from build123d import *

# Parameters (mm, degrees)
BASE_FLANGE1_DEPTH            = 1
EDGE_FLANGE1_STRIP_W          = 6
EDGE_FLANGE1_STRIP_H          = 1
EDGE_FLANGE1_STRIP_CUT_DEPTH  = 100
EDGE_FLANGE1_RELIEF_W         = 6.5
EDGE_FLANGE1_RELIEF_H         = 0.5
EDGE_FLANGE1_RELIEF_CUT_DEPTH = 1
EDGE_FLANGE1_DEPTH            = 100
EDGE_FLANGE1_PROFILE_W        = 100
EDGE_FLANGE1_PROFILE_H        = 19
EDGE_FLANGE1_PROFILE_R        = 1.5
EDGE_FLANGE1_FLAT_DEPTH       = 1
EDGE_FLANGE2_START            = 29.5
EDGE_FLANGE2_DEPTH            = 61
EDGE_FLANGE2_2_DEPTH          = 0.5
EDGE_FLANGE2_START_2          = 90
EDGE_FLANGE2_3_DEPTH          = 0.5
EDGE_FLANGE2_START_3          = 30
EDGE_FLANGE2_4_DEPTH          = 60
EDGE_FLANGE2_5_OUTLINE_R      = 1.5
EDGE_FLANGE2_5_DEPTH          = 1


with BuildPart() as part:
    # Base-Flange1: sheet metal written as solids
    # Sketch1 → Base-Flange1 (new body)
    with BuildSketch(Plane.XY):
        with BuildLine():
            Line((0, 0), (0, 350))
            Line((0, 350), (0, 375))
            ThreePointArc((0, 375), (-13.854151002, 365.75), (-27.708302005, 375))
            ThreePointArc((-27.708302005, 375), (-5.863059775, 415.921497754), (30, 386.5))
            Line((30, 386.5), (30, 346.5))
            Line((30, 346.5), (600, 280))
            Line((600, 280), (600, 0))
            Line((600, 0), (0, 0))
        make_face()
    extrude(amount=-BASE_FLANGE1_DEPTH)

    # Edge-Flange1: sheet metal written as solids
    # Edge-Flange1 strip (on a plane across the edge) → Edge-Flange1 strip cut (cut)
    with BuildSketch(Plane.YZ.offset(450)):
        with Locations((-1, -0.5)):
            Rectangle(EDGE_FLANGE1_STRIP_W, EDGE_FLANGE1_STRIP_H)
    edge_flange1_strip_cut = extrude(amount=EDGE_FLANGE1_STRIP_CUT_DEPTH, mode=Mode.SUBTRACT)

    # Edge-Flange1 relief (on the sheet) → Edge-Flange1 relief cut (cut)
    with BuildSketch(Plane(origin=(450, 2, 0), x_dir=(0, 1, 0), z_dir=(0, 0, 1))):
        with Locations((-2.75, 0.25)):
            Rectangle(EDGE_FLANGE1_RELIEF_W, EDGE_FLANGE1_RELIEF_H)
        with Locations((-2.75, -100.25)):
            Rectangle(EDGE_FLANGE1_RELIEF_W, EDGE_FLANGE1_RELIEF_H)
    edge_flange1_relief_cut = extrude(amount=-EDGE_FLANGE1_RELIEF_CUT_DEPTH, mode=Mode.SUBTRACT)

    # Edge-Flange1 bend section (on a plane across the edge) → Edge-Flange1 (add)
    with BuildSketch(Plane.YZ.offset(450)):
        with BuildLine():
            Line((0, 1), (1, 1))
            ThreePointArc((1, 1), (1.292893219, 0.292893219), (2, 0))
            Line((2, 0), (2, -1))
            ThreePointArc((2, -1), (0.585786438, -0.414213562), (0, 1))
        make_face()
    edge_flange1 = extrude(amount=EDGE_FLANGE1_DEPTH)

    # Edge-Flange1 profile (on flange) → Edge-Flange1 flat (add)
    with BuildSketch(Plane(origin=(0, 0, 0), x_dir=(-1, 0, 0), z_dir=(0, 1, 0))):
        with Locations((-500, 10.5)):
            Rectangle(EDGE_FLANGE1_PROFILE_W, EDGE_FLANGE1_PROFILE_H)
        with Locations((-535, 10)):
            Circle(EDGE_FLANGE1_PROFILE_R, mode=Mode.SUBTRACT)
        with Locations((-465, 10)):
            Circle(EDGE_FLANGE1_PROFILE_R, mode=Mode.SUBTRACT)
        with Locations((-500, 10)):
            Circle(EDGE_FLANGE1_PROFILE_R, mode=Mode.SUBTRACT)
    edge_flange1_flat = extrude(amount=EDGE_FLANGE1_FLAT_DEPTH)

    # Mirror1: Edge-Flange1 strip cut, Edge-Flange1 relief cut, Edge-Flange1, Edge-Flange1 flat across plane
    add(edge_flange1_strip_cut.mirror(Plane(origin=(300, 0, 0), x_dir=(0, 0, 1), z_dir=(1, 0, 0))), mode=Mode.SUBTRACT)
    add(edge_flange1_relief_cut.mirror(Plane(origin=(300, 0, 0), x_dir=(0, 0, 1), z_dir=(1, 0, 0))), mode=Mode.SUBTRACT)
    add(edge_flange1.mirror(Plane(origin=(300, 0, 0), x_dir=(0, 0, 1), z_dir=(1, 0, 0))))
    add(edge_flange1_flat.mirror(Plane(origin=(300, 0, 0), x_dir=(0, 0, 1), z_dir=(1, 0, 0))))

    # Edge-Flange2: read off the stored shape, not the designer's step
    # Edge-Flange2 outline → Edge-Flange2 (cut)
    with BuildSketch(Plane(origin=(0, 0, 0), x_dir=(1, 0, 0), z_dir=(0, 1, 0)).offset(EDGE_FLANGE2_START)):
        with BuildLine():
            ThreePointArc((0.363077531, 0), (1.095128339, 0.732050808), (2.095128339, 1))
            Line((2.095128339, 1), (0, 1))
            Line((0, 1), (0, 0))
            Line((0, 0), (0.363077531, 0))
        make_face()
    edge_flange2 = extrude(amount=EDGE_FLANGE2_DEPTH, mode=Mode.SUBTRACT)

    # Edge-Flange2 2 outline → Edge-Flange2 2 (cut)
    with BuildSketch(Plane(origin=(0, 0, 0), x_dir=(1, 0, 0), z_dir=(0, 1, 0)).offset(EDGE_FLANGE2_START)):
        with BuildLine():
            Line((2.595128339, 0), (2.595128339, 1))
            Line((2.595128339, 1), (2.095128339, 1))
            ThreePointArc((2.095128339, 1), (1.095128339, 0.732050808), (0.363077531, 0))
            Line((0.363077531, 0), (2.595128339, 0))
        make_face()
    edge_flange2_2 = extrude(amount=EDGE_FLANGE2_2_DEPTH, mode=Mode.SUBTRACT)

    # Edge-Flange2 3 outline → Edge-Flange2 3 (cut)
    with BuildSketch(Plane(origin=(0, 0, 0), x_dir=(1, 0, 0), z_dir=(0, 1, 0)).offset(EDGE_FLANGE2_START_2)):
        with BuildLine():
            Line((2.595128339, 0), (2.595128339, 1))
            Line((2.595128339, 1), (2.095128339, 1))
            ThreePointArc((2.095128339, 1), (1.095128339, 0.732050808), (0.363077531, 0))
            Line((0.363077531, 0), (2.595128339, 0))
        make_face()
    edge_flange2_3 = extrude(amount=EDGE_FLANGE2_3_DEPTH, mode=Mode.SUBTRACT)

    # Edge-Flange2 4 outline → Edge-Flange2 4 (add)
    with BuildSketch(Plane(origin=(0, 0, 0), x_dir=(1, 0, 0), z_dir=(0, 1, 0)).offset(EDGE_FLANGE2_START_3)):
        with BuildLine():
            ThreePointArc((1.098933641, -1.087155743), (1.357851002, -0.324409792), (2.095128339, 0))
            Line((2.095128339, 0), (0.363077531, 0))
            ThreePointArc((0.363077531, 0), (0.142536324, -0.567120772), (0.102738942, -1.174311485))
            Line((0.102738942, -1.174311485), (1.750739994, -20.011049705))
            Line((1.750739994, -20.011049705), (2.746934692, -19.923893962))
            Line((2.746934692, -19.923893962), (1.098933641, -1.087155743))
        make_face()
    edge_flange2_4 = extrude(amount=EDGE_FLANGE2_4_DEPTH)

    # Edge-Flange2 5 outline → Edge-Flange2 5 (cut)
    with BuildSketch(Plane(origin=(0, 0, 0), x_dir=(0, 1, 0), z_dir=(0.9961946980917459, 0, -0.0871557427476548))):
        with Locations((80, 10.087488664)):
            Circle(EDGE_FLANGE2_5_OUTLINE_R)
        with Locations((60, 10.087488664)):
            Circle(EDGE_FLANGE2_5_OUTLINE_R)
        with Locations((40, 10.087488664)):
            Circle(EDGE_FLANGE2_5_OUTLINE_R)
    edge_flange2_5 = extrude(amount=EDGE_FLANGE2_5_DEPTH, mode=Mode.SUBTRACT)

    # Mirror2: Edge-Flange2, Edge-Flange2 2, Edge-Flange2 3, Edge-Flange2 4, Edge-Flange2 5 across plane
    add(edge_flange2.mirror(Plane.ZX.offset(161.81)), mode=Mode.SUBTRACT)
    add(edge_flange2_2.mirror(Plane.ZX.offset(161.81)), mode=Mode.SUBTRACT)
    add(edge_flange2_3.mirror(Plane.ZX.offset(161.81)), mode=Mode.SUBTRACT)
    add(edge_flange2_4.mirror(Plane.ZX.offset(161.81)))
    add(edge_flange2_5.mirror(Plane.ZX.offset(161.81)), mode=Mode.SUBTRACT)


solid = part.part
Read the model definition and answer for the solid it produces. Units are mm, in the model's axes. A direction names the side the tool comes from. Round coordinates to 2 decimals unless told otherwise and drop trailing zeros. Write each loop counter-clockwise with the first axis right and the second up, starting at its lowest first coordinate (ties: lowest second). Pieces come first, ordered by that corner, then holes. Notation, with made-up numbers: (48.25, 14) - (61.25, 14) arc R9 ccw to (61.25, 30) - close; hole circle Ø2 at (65, 81). An arc over 180 degrees is marked (long way). Use a Markdown table: item, result.
(1) Each of these flat-tipped pins is pushed along its axis until it touches: pin 1 Ø1.1 at (y, z) = (1, -0.5) entering from -X; pin 2 Ø2 at (x, z) = (309, 2) entering from +Y; pin 3 Ø3.5 at (x, z) = (100, 10) entering from +Y; pin 4 Ø0.6 at (y, z) = (233.5, -0.5) entering from -X. Where does it stop, or does it pass through?
Reported:
| item | result |
|---|---|
| pin 1 | x = 0 |
| pin 2 | through |
| pin 3 | y = 1 |
| pin 4 | x = 0.51 |
(2) The part is cut by section A-A (z = 14.75). Write down the section's boundary in (x, y), then the cut area to 3 significant figures.
Reported:
| item | result |
|---|---|
| outline | (1.29, 30) - (2.29, 30) - (2.29, 90) - (1.29, 90) - close; (1.29, 233.62) - (2.29, 233.62) - (2.29, 293.62) - (1.29, 293.62) - close; (50, 0) - (150, 0) - (150, 1) - (50, 1) - close; (450, 0) - (550, 0) - (550, 1) - (450, 1) - close |
| area | 320 mm2 |
(3) Straight lines are drawn through the part: line 1 along Z through (x, y) = (500, 0.2); line 2 along Z through (x, y) = (341, 245); line 3 along Y through (x, z) = (513, 1). For each, find the intervals that lie inside material, in ascending order. Write a range as [from, to].
Reported:
| item | result |
|---|---|
| line 1 | [0.13, 8.5], [11.5, 20] |
| line 2 | [-1, 0] |
| line 3 | [0, 1] |
(4) The mould has two halves that part along Z. Classify faces 4 (the flat face through (289, 165, -1)), 5 (the flat face through (2.118, 264.04, 12.73)), 6 (the flat face through (501, 0, 13)), 7 (the flat face through (0.732, 264.04, 8.368)): released by +Z, released by -Z, zero draft, split by the parting line, or undercut.
Reported:
| item | result |
|---|---|
| face 4 | released by -Z |
| face 5 | undercut |
| face 6 | zero draft |
| face 7 | released by +Z |
(5) The part is cut by section D-D (x = 198). Write down the section's boundary in (y, z), then the cut area to 3 significant figures.
Reported:
| item | result |
|---|---|
| outline | (0, -1) - (326.9, -1) - (326.9, 0) - (0, 0) - close |
| area | 327 mm2 |
(6) The part is cut by section B-B (x = 474.5). Write down the section's boundary in (y, z).
Reported:
| item | result |
|---|---|
| outline | (0, 1) arc R2 ccw to (2, -1) - (294.64, -1) - (294.64, 0) - (2, 0) arc R1 cw to (1, 1) - (1, 20) - (0, 20) - close |
(7) The part is cut by section C-C (y = 156.5). Write down the section's boundary in (x, z).
Reported:
| item | result |
|---|---|
| outline | (0, -1) - (600, -1) - (600, 0) - (0, 0) - close |
(8) Which of the six approach directions +Z, -Z, +X, -X, +Y, -Y give full straight-line access (tool end or side, diameter ignored) to faces 1 (the flat face through (2.118, 59.58, 12.73)), 2 (the flat face through (99, 1, 13)), 3 (the flat face through (0.732, 59.58, 8.368))?
Reported:
| item | result |
|---|---|
| face 1 | +X, +Y, -Y |
| face 2 | +Z, +X, -X, +Y |
| face 3 | +Z, -X, +Y, -Y |
